Job drawing, mm, ordinate dimensions from the low corner. One solid piece. A direction names the side the tool comes from. Give positions to 0.01 mm unless a question says otherwise; leave off trailing zeros. Loops run counter-clockwise (first coordinate to the right, second up) from the corner with the lowest first, then second, coordinate; pieces in that order, holes last. Notation, with made-up numbers: (-0.75, 27) - (33.25, 27) arc R34 cw to (33.25, 66) - close; hole circle Ø9 at (64.25, 87.25). An arc over 180 degrees is marked (long way). Use a Markdown table: item, result.
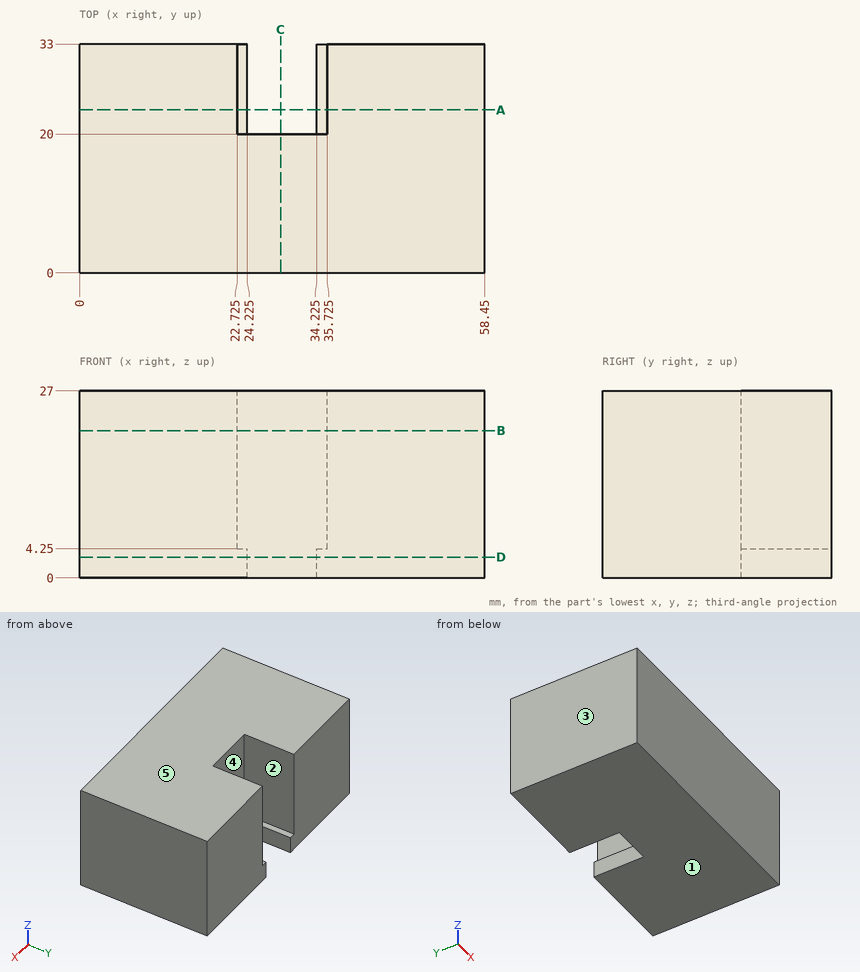
(1) Drill centre lines: probe 1 along X at (y, z) = (31.5, 3.75) (3 decimals); probe 2 along X at (y, z) = (26, 17) (3 decimals); probe 3 along Y at (x, z) = (23.5, 14.25). Where is each one in solid material? Low to high. Write a range as [from, to].
Computed:
| item | result |
|---|---|
| probe 1 | [0, 24.225], [34.225, 58.45] |
| probe 2 | [0, 22.725], [35.725, 58.45] |
| probe 3 | [0, 20] |
(2) Pin check, flat tips, straight feed: P1, Ø4, axis at x = 27.5, z = 12, coming from the +Y side; P2, Ø1.2, axis at x = 35, y = 27.5, coming from the +Z side. Stop position of each tip, or through.
Computed:
| item | result |
|---|---|
| P1 | y = 20 |
| P2 | z = 4.25 |
(3) Mould opens along X. For the marked faces 3, 4 and 5 say: pulls with the +X half, pulls with the -X half, needs draft (parallel to the pull), parting line crosses it, or undercut.
Computed:
| item | result |
|---|---|
| face 3 | pulls with the -X half |
| face 4 | undercut |
| face 5 | needs draft |
(4) Slice it at B-B, the plane z = 21.25. Write the cut outline in (x, y) (3 decimals), plus the area to 3 significant figures.
Computed:
| item | result |
|---|---|
| outline | (0, 0) - (58.45, 0) - (58.45, 33) - (35.725, 33) - (35.725, 20) - (22.725, 20) - (22.725, 33) - (0, 33) - close |
| area | 1,760 mm² |
(5) Slice it at A-A, the plane y = 23.5. Write the cut outline in (x, z) (3 decimals), plus the area to 3 significant figures.
Computed:
| item | result |
|---|---|
| outline | (0, 0) - (24.225, 0) - (24.225, 4.25) - (22.725, 4.25) - (22.725, 27) - (0, 27) - close; (34.225, 0) - (58.45, 0) - (58.45, 27) - (35.725, 27) - (35.725, 4.25) - (34.225, 4.25) - close |
| area | 1,240 mm² |
(6) Slice it at D-D, the plane z = 3. Write the cut outline in (x, y) (3 decimals).
Computed:
| item | result |
|---|---|
| outline | (0, 0) - (58.45, 0) - (58.45, 33) - (34.225, 33) - (34.225, 20) - (24.225, 20) - (24.225, 33) - (0, 33) - close |
(7) 3-axis set-ups, long thin cutter, end or side, ignore diameter. For the marked faces 1 and 2: which of +Z, -Z, +X, -X, +Y, -Y reach the whole face in a straight line?
Computed:
| item | result |
|---|---|
| face 1 | -Z, +X, -X, +Y, -Y |
| face 2 | +Z, +Y |
(8) Slice it at C-C, the plane x = 29. Write the cut outline in (y, z), plus the area to 3 significant figures.
Computed:
| item | result |
|---|---|
| outline | (0, 0) - (20, 0) - (20, 27) - (0, 27) - close |
| area | 540 mm² |
